Build history of the part. All positions in model axes, mm. Face numbers are marked on the shaded views. A direction names the side the tool comes from. Give positions to 0.01 mm unless a question says otherwise; leave off trailing zeros. Order: outer loops, then holes, each group sorted by start corner. A loop starts at its lowest first (then second) coordinate and runs counter-clockwise, first axis right, second up. Notation, with made-up numbers: (75, 58.25) - (120, 58.25) arc R19 ccw to (120, 91.25) - close; hole circle Ø6 at (54, 18.5). An arc over 180 degrees is marked (long way). Answer in a Markdown table with one row per item.
```python
from build123d import *

# Parameters (mm, degrees)
SKETCH1_W               = 139.7
SKETCH1_H               = 139.7
SKETCH1_W_2             = 101.6
SKETCH1_H_2             = 101.6
EXTRUDE_THIN1_DEPTH     = 152.4
CUT_EXTRUDE2_START      = -50.8
SKETCH3_W               = 19.05
SKETCH3_H               = 101.6
CUT_EXTRUDE2_DEPTH      = 50.8
BOSS_EXTRUDE2_DEPTH     = 76.2
SKETCH6_W               = 69.85
SKETCH6_H               = 101.6
CUT_EXTRUDE3_DEPTH      = 223.34069578
SKETCH8_R               = 6.35
CUT_EXTRUDE4_DEPTH      = 254.125369136
SKETCH9_W               = 215.9
SKETCH9_H               = 152.4
CUT_EXTRUDE5_DEPTH      = 304.76371755
CUT_EXTRUDE6_DEPTH      = 355.386895074
CUT_EXTRUDE6_DEPTH_BACK = 355.386895074
SKETCH11_R              = 19.05


with BuildPart() as part:
    # Sketch1 → Extrude-Thin1 (new body)
    with BuildSketch(Plane(origin=(0, 0, 0), x_dir=(1, 0, 0), z_dir=(0, 1, 0))):
        Rectangle(SKETCH1_W, SKETCH1_H)
        Rectangle(SKETCH1_W_2, SKETCH1_H_2, mode=Mode.SUBTRACT)
    extrude(amount=EXTRUDE_THIN1_DEPTH)

    # Sketch3 → Cut-Extrude2 (cut)
    with BuildSketch(Plane.XZ.offset(CUT_EXTRUDE2_START)):
        with Locations((-60.325, 0)):
            Rectangle(SKETCH3_W, SKETCH3_H)
    cut_extrude2 = extrude(amount=CUT_EXTRUDE2_DEPTH, mode=Mode.SUBTRACT)

    # Sketch5 → Boss-Extrude2 (add)
    with BuildSketch(Plane.ZY.offset(69.85)):
        Polygon((-50.8, 50.8), (50.8, 50.8), (50.8, 0), (69.85, 0), (69.85, 152.4), (-69.85, 152.4), (-69.85, 0), (-50.8, 0), align=None)
    boss_extrude2 = extrude(amount=BOSS_EXTRUDE2_DEPTH)

    # Sketch6 → Cut-Extrude3 (cut, through all)
    with BuildSketch(Plane(origin=(0, 152.4, 0), x_dir=(1, 0, 0), z_dir=(0, 1, 0))):
        with Locations((-98.425, 0)):
            Rectangle(SKETCH6_W, SKETCH6_H)
    cut_extrude3 = extrude(amount=-CUT_EXTRUDE3_DEPTH, mode=Mode.SUBTRACT)

    # Sketch8 → Cut-Extrude4 (cut, through all)
    with BuildSketch(Plane.XY.offset(69.85)):
        with Locations((-98.298, 25.4)):
            Circle(SKETCH8_R)
    cut_extrude4 = extrude(amount=-CUT_EXTRUDE4_DEPTH, mode=Mode.SUBTRACT)

    # Mirror3: Cut-Extrude2, Boss-Extrude2, Cut-Extrude3, Cut-Extrude4 across plane
    add(cut_extrude2.mirror(Plane(origin=(0, 0, 0), x_dir=(-0.7071067811865476, 0, 0.7071067811865476), z_dir=(-0.7071067811865477, 0, -0.7071067811865475))), mode=Mode.SUBTRACT)
    add(boss_extrude2.mirror(Plane(origin=(0, 0, 0), x_dir=(-0.7071067811865476, 0, 0.7071067811865476), z_dir=(-0.7071067811865477, 0, -0.7071067811865475))))
    add(cut_extrude3.mirror(Plane(origin=(0, 0, 0), x_dir=(-0.7071067811865476, 0, 0.7071067811865476), z_dir=(-0.7071067811865477, 0, -0.7071067811865475))), mode=Mode.SUBTRACT)
    add(cut_extrude4.mirror(Plane(origin=(0, 0, 0), x_dir=(-0.7071067811865476, 0, 0.7071067811865476), z_dir=(-0.7071067811865477, 0, -0.7071067811865475))), mode=Mode.SUBTRACT)


with BuildPart() as body_2:
    # Mirror5: mirrored copy
    add(part.part.mirror(Plane(origin=(72.39, 0, 0), x_dir=(0, 0, 1), z_dir=(1, 0, 0))))

    # Sketch11 → Cut-Extrude6 (cut, two sides: drawn at the far end of the back side and taken through both)
    with BuildSketch(Plane.XY.offset(63.5).offset(-CUT_EXTRUDE6_DEPTH_BACK)):
        with Locations((144.78, 114.3)):
            Circle(SKETCH11_R)
    extrude(amount=CUT_EXTRUDE6_DEPTH + CUT_EXTRUDE6_DEPTH_BACK, mode=Mode.SUBTRACT)


with BuildPart() as part_1:
    add(part.part)

    # Sketch9 → Cut-Extrude5 (cut, through all)
    with BuildSketch(Plane(origin=(72.39, 0, 0), x_dir=(0, 0, -1), z_dir=(1, 0, 0))):
        with Locations((-38.1, 76.2)):
            Rectangle(SKETCH9_W, SKETCH9_H)
    extrude(amount=-CUT_EXTRUDE5_DEPTH, mode=Mode.SUBTRACT)


solid = body_2.part
```
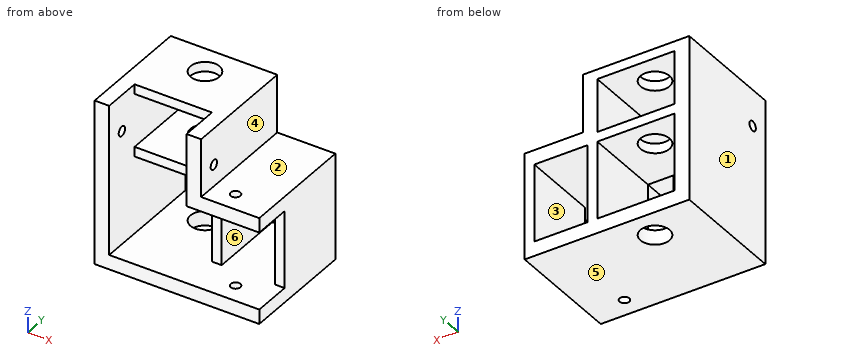
1. Probe line 1 (X direction, y = 66.5, z = 6.5); line 2 (Z direction, x = 187, y = 140.5); line 3 (Z direction, x = 219.5, y = 10). List the from-to ranges inside material, lowest first.
Check result:
| item | result |
|---|---|
| line 1 | x = 74.93 to 93.98, 195.58 to 208.28, 278.13 to 290.83 |
| line 2 | z = -69.85 to -50.8, 50.8 to 63.5, 133.35 to 146.05 |
| line 3 | z = -69.85 to -50.8, 50.8 to 69.85 |
2. Drop flat-ended pins along their axis: P1, Ø4, axis at y = 68.5, z = 120, coming from the +X side; P2, Ø20.5, axis at y = 25.4, z = 98.298, coming from the -X side; P3, Ø6.5, axis at x = 284.5, z = -18, coming from the -Y side; P4, Ø1, axis at y = 19.5, z = -11, coming from the +X side. Give the stop position or say it passes through.
Check result:
| item | result |
|---|---|
| P1 | stops at x = 214.63 |
| P2 | stops at x = 74.93 |
| P3 | stops at y = 50.8 |
| P4 | stops at x = 93.98 |
3. Cut at A-A on y = 114.3. Count the separate pieces of the cut face and the enclosed holes in it, and give its area (3 significant figures).
Check result:
| item | result |
|---|---|
| separate pieces | 2 |
| enclosed holes | 1 |
| area | 14,600 mm² |
4. Cut at B-B on z = 109.5. Write the cut outline in (x, y).
Check result:
| item | result |
|---|---|
| outline | (74.93, 0) - (93.98, 0) - (93.98, 152.4) - (74.93, 152.4) - close; (195.58, 0) - (214.63, 0) - (214.63, 152.4) - (195.58, 152.4) - close |
5. Cut at C-C on x = 121.5. Write the cut outline in (y, z), and give its area (3 significant figures).
Check result:
| item | result |
|---|---|
| outline | (0, -69.85) - (152.4, -69.85) - (152.4, -50.8) - (0, -50.8) - close; (50.8, 50.8) - (152.4, 50.8) - (152.4, 63.5) - (50.8, 63.5) - close; (50.8, 133.35) - (152.4, 133.35) - (152.4, 146.05) - (50.8, 146.05) - close |
| area | 5,480 mm² |
6. Which spindle directions (+Z, -Z, +X, -X, +Y, -Y) get a long thin tool onto all of the face, cutting with end or side? Do the marked faces 1, 2 and 3. Say none if no direction does.
Check result:
| item | result |
|---|---|
| face 1 | +Z, -Z, -X, +Y, -Y |
| face 2 | +Z, +X, +Y, -Y |
| face 3 | +Y, -Y |
7. Cut at D-D on x = 144.78. Write the cut outline in (y, z), and give its area (3 significant figures).
Check result:
| item | result |
|---|---|
| outline | (0, -69.85) - (95.25, -69.85) - (95.25, -50.8) - (0, -50.8) - close; (50.8, 50.8) - (95.25, 50.8) - (95.25, 63.5) - (50.8, 63.5) - close; (50.8, 133.35) - (95.25, 133.35) - (95.25, 146.05) - (50.8, 146.05) - close; (133.35, -69.85) - (152.4, -69.85) - (152.4, -50.8) - (133.35, -50.8) - close; (133.35, 50.8) - (152.4, 50.8) - (152.4, 63.5) - (133.35, 63.5) - close; (133.35, 133.35) - (152.4, 133.35) - (152.4, 146.05) - (133.35, 146.05) - close |
| area | 3,790 mm² |
8. Two-plate mould, pull along Z, no slides. Class the marked faces 4, 5 and 6: +Z half, -Z half, draft (parallel to the pull), parting line (faces both ways), or undercut.
Check result:
| item | result |
|---|---|
| face 4 | draft |
| face 5 | -Z half |
| face 6 | undercut |
